Read the model definition and answer for the solid it produces. Units are mm, in the model's axes. A direction names the side the tool comes from. Coordinates: 2 decimals unless noted, no trailing zeros. Order: outer loops, then holes, each group sorted by start corner. A loop starts at its lowest first (then second) coordinate and runs counter-clockwise, first axis right, second up. Notation, with made-up numbers: (-31, -28) - (13, -28) arc R16 cw to (13, -19) - close; hole circle Ø3 at (47, -21.75). An arc over 180 degrees is marked (long way). Answer as a JSON object with one key per item and string values. Group by question number.
from build123d import *

# Parameters (mm, degrees)
SKETCH1_W           = 135
SKETCH1_H           = 40
SKETCH1_R           = 2
BOSS_EXTRUDE1_DEPTH = 4
SKETCH3_W           = 3
SKETCH3_H           = 40
BOSS_EXTRUDE3_DEPTH = 200


with BuildPart() as part:
    # Sketch1 → Boss-Extrude1 (new body)
    with BuildSketch(Plane(origin=(0, 0, 0), x_dir=(1, 0, 0), z_dir=(0, 1, 0))):
        Rectangle(SKETCH1_W, SKETCH1_H)
        with Locations(Location((-21.5, 14, 0), (0, 0, 270))):
            Circle(SKETCH1_R, mode=Mode.SUBTRACT)
        with Locations(Location((-21.5, -14, 0), (0, 0, 270))):
            Circle(SKETCH1_R, mode=Mode.SUBTRACT)
        with Locations(Location((-61.5, -14, 0), (0, 0, 270))):
            Circle(SKETCH1_R, mode=Mode.SUBTRACT)
        with Locations(Location((-61.5, 14, 0), (0, 0, 270))):
            Circle(SKETCH1_R, mode=Mode.SUBTRACT)
    extrude(amount=BOSS_EXTRUDE1_DEPTH)

    # Sketch3 → Boss-Extrude3 (add)
    with BuildSketch(Plane.XZ):
        with Locations((66, 0)):
            Rectangle(SKETCH3_W, SKETCH3_H)
    extrude(amount=BOSS_EXTRUDE3_DEPTH)


solid = part.part
1. A cutting plane is placed at D-D on z = 9.5. Write down the section's boundary in (x, y).
2. For a pull along Z with two mould halves and no side action, classify faces 3 (the flat face through (-2, 0, 0)), 4 (the flat face through (65, -52, 20)), 5 (the cylindrical face through (-59.517, 1.972, 13.74)) as pulls with the +Z half, pulls with the -Z half, needs draft (parallel to the pull), parting line crosses it, or undercut.
3. A cutting plane is placed at C-C on y = -170. Write down the section's boundary in (x, z).
4. Given pin 1 (4.5 mm diameter, centred on x = -21.5, z = 14, fed in from -Y); pin 2 (2.5 mm diameter, centred on x = -61.5, z = -14, fed in from -Y), each flat-ended and moving along its own axis, determine where each tip first touches the part or whether it passes through.
5. A cutting plane is placed at B-B on x = -21.5. Write down the section's boundary in (y, z), and give its area (3 significant figures).
6. Straight lines are drawn through the part: L1, parallel to X at y = 2.2, z = 14; L2, parallel to Y at x = 39.5, z = -6; L3, parallel to Z at x = -21, y = 1. For each, find the intervals that lie inside material, in ascending order.
7. For faces 1 (the flat face through (64.5, -99, 0)), 2 (the flat face through (-67.5, 2, 0)), determine the directions among +Z, -Z, +X, -X, +Y, -Y from which every point of the face is accessible in a straight line to the end or side of a thin tool.
8. A cutting plane is placed at A-A on z = -14. Write down the section's boundary in (x, y), and give its area (3 significant figures).
Derived:
{
 "1": {"outline": "(-67.5, 0) - (64.5, 0) - (64.5, -200) - (67.5, -200) - (67.5, 4) - (-67.5, 4) - close"},
 "2": {"face 3": "needs draft", "face 4": "pulls with the +Z half", "face 5": "undercut"},
 "3": {"outline": "(64.5, -20) - (67.5, -20) - (67.5, 20) - (64.5, 20) - close"},
 "4": {"pin 1": "stops at y = 0", "pin 2": "passes through"},
 "5": {"outline": "(0, -20) - (4, -20) - (4, -16) - (0, -16) - close; (0, -12) - (4, -12) - (4, 12) - (0, 12) - close; (0, 16) - (4, 16) - (4, 20) - (0, 20) - close", "area": "128 mm2"},
 "6": {"L1": "x = -67.5 to -63.5, -59.5 to -23.5, -19.5 to 67.5", "L2": "y = 0 to 4", "L3": "z = -20 to -15.94, -12.06 to 12.06, 15.94 to 20"},
 "7": {"face 1": "+Z, -Z, -X, -Y", "face 2": "+Z, -Z, -X, +Y, -Y"},
 "8": {"outline": "(-67.5, 0) - (-63.5, 0) - (-63.5, 4) - (-67.5, 4) - close; (-59.5, 0) - (-23.5, 0) - (-23.5, 4) - (-59.5, 4) - close; (-19.5, 0) - (64.5, 0) - (64.5, -200) - (67.5, -200) - (67.5, 4) - (-19.5, 4) - close", "area": "1,110 mm2"}
}
